Design review of the part built by this model. Coordinates are the model's own, in mm. A direction names the side the tool comes from. Coordinates: 2 decimals unless noted, no trailing zeros. Loops run counter-clockwise (first coordinate to the right, second up) from the corner with the lowest first, then second, coordinate; pieces in that order, holes last. Notation, with made-up numbers: (-35.75, 79) - (-19.75, 79) arc R24 cw to (-19.75, 102) - close; hole circle Ø9 at (30, 56). An arc over 180 degrees is marked (long way). Return JSON: item names as keys, results as strings. Group by question number.
from build123d import *

# Parameters (mm, degrees)
BOSS_EXTRUDE1_DEPTH = 2
SKETCH4_R           = 1.6
CUT_EXTRUDE4_DEPTH  = 414.677410551
SKETCH3_R           = 2.5
SKETCH3_R_2         = 1.5
BOSS_EXTRUDE3_DEPTH = 1
SKETCH5_W           = 24
SKETCH5_H           = 28
BOSS_EXTRUDE2_DEPTH = 7
SKETCH2_W           = 19
SKETCH2_H           = 24.51763809
CUT_EXTRUDE5_DEPTH  = 9
BOSS_EXTRUDE4_REACH = 375.267
SKETCH8_W           = 28
SKETCH8_H           = 24
SKETCH9_R           = 1.5
CUT_EXTRUDE7_DEPTH  = 414.770467772


with BuildPart() as part:
    # Sketch1 → Boss-Extrude1 (new body)
    with BuildSketch(Plane.XY):
        with BuildLine():
            Line((0, 2), (288, 2))
            ThreePointArc((288, 2), (289.414213562, 1.414213562), (290, 0))
            Line((290, 0), (290, -293))
            ThreePointArc((290, -293), (289.414213562, -294.414213562), (288, -295))
            Line((288, -295), (0, -295))
            ThreePointArc((0, -295), (-1.414213562, -294.414213562), (-2, -293))
            Line((-2, -293), (-2, 0))
            ThreePointArc((-2, 0), (-1.414213562, 1.414213562), (0, 2))
        make_face()
    extrude(amount=BOSS_EXTRUDE1_DEPTH)

    # Sketch4 → Cut-Extrude4 (cut, through all)
    with BuildSketch(Plane(origin=(0, 0, 0), x_dir=(-1, 0, 0), z_dir=(0, 0, -1))):
        with Locations((-271, -256)):
            Circle(SKETCH4_R)
        with Locations(Location((-271, -37, 0), (0, 0, 180))):
            Circle(SKETCH4_R)
        with Locations(Location((-17, -256, 0), (0, 0, 180))):
            Circle(SKETCH4_R)
        with Locations((-17, -37)):
            Circle(SKETCH4_R)
    extrude(amount=-CUT_EXTRUDE4_DEPTH, mode=Mode.SUBTRACT)

    # Sketch3 → Boss-Extrude3 (add)
    # profile 1 of 4: a face of its own
    with BuildSketch(Plane(origin=(0, 0, 2), x_dir=(-1, 0, 0), z_dir=(0, 0, -1))):
        with Locations((-271, -37)):
            Circle(SKETCH3_R)
        with Locations((-271, -37)):
            Circle(SKETCH3_R_2, mode=Mode.SUBTRACT)
    # profile 2 of 4: a face of its own
    with BuildSketch(Plane(origin=(0, 0, 2), x_dir=(-1, 0, 0), z_dir=(0, 0, -1))):
        with Locations(Location((-17, -37, 0), (0, 0, 180))):
            Circle(SKETCH3_R)
        with Locations(Location((-17, -37, 0), (0, 0, 180))):
            Circle(SKETCH3_R_2, mode=Mode.SUBTRACT)
    # profile 3 of 4: a face of its own
    with BuildSketch(Plane(origin=(0, 0, 2), x_dir=(-1, 0, 0), z_dir=(0, 0, -1))):
        with Locations((-17, -256)):
            Circle(SKETCH3_R)
        with Locations((-17, -256)):
            Circle(SKETCH3_R_2, mode=Mode.SUBTRACT)
    # profile 4 of 4: a face of its own
    with BuildSketch(Plane(origin=(0, 0, 2), x_dir=(-1, 0, 0), z_dir=(0, 0, -1))):
        with Locations(Location((-271, -256, 0), (0, 0, 180))):
            Circle(SKETCH3_R)
        with Locations(Location((-271, -256, 0), (0, 0, 180))):
            Circle(SKETCH3_R_2, mode=Mode.SUBTRACT)
    extrude(amount=-BOSS_EXTRUDE3_DEPTH)

    # Sketch5 → Boss-Extrude2 (add)
    with BuildSketch(Plane.XY.offset(2)):
        with Locations((273, -68.5)):
            Rectangle(SKETCH5_W, SKETCH5_H)
        with Locations((273, -224.5)):
            Rectangle(SKETCH5_W, SKETCH5_H)
    extrude(amount=BOSS_EXTRUDE2_DEPTH)

    # Sketch2 → Cut-Extrude5 (cut)
    with BuildSketch(Plane(origin=(19.360490202, 0, -72.51763809), x_dir=(0, -1, 0), z_dir=(-0.25881904510252135, 0, 0.9659258262890681))):
        Polygon((234, 285.704276061), (215, 285.704276061), (215.5, 261.186637971), (233.5, 261.186637971), align=None)
        with Locations((68.5, 273.445457016)):
            Rectangle(SKETCH2_W, SKETCH2_H)
    extrude(amount=CUT_EXTRUDE5_DEPTH, mode=Mode.SUBTRACT)

    # Sketch8 → Boss-Extrude4 (add, up to next)
    with BuildSketch(Plane(origin=(103.407277926, 0, -123.235994969), x_dir=(0, -1, 0), z_dir=(-0.6427876096865406, 0, 0.7660444431189771)), mode=Mode.PRIVATE) as boss_extrude4_sk1:
        with Locations((68.5, 193.722688141)):
            Rectangle(SKETCH8_W, SKETCH8_H)
    boss_extrude4_tool1 = extrude(boss_extrude4_sk1.sketch, amount=-BOSS_EXTRUDE4_REACH, mode=Mode.PRIVATE) - part.part
    # Sketch8 → Boss-Extrude4 (add, up to next)
    with BuildSketch(Plane(origin=(103.407277926, 0, -123.235994969), x_dir=(0, -1, 0), z_dir=(-0.6427876096865406, 0, 0.7660444431189771)), mode=Mode.PRIVATE) as boss_extrude4_sk2:
        with Locations((224.5, 193.722688141)):
            Rectangle(SKETCH8_W, SKETCH8_H)
    boss_extrude4_tool2 = extrude(boss_extrude4_sk2.sketch, amount=-BOSS_EXTRUDE4_REACH, mode=Mode.PRIVATE) - part.part
    add(boss_extrude4_tool1.solids().sort_by_distance((251.807467, -68.5, 1.286549))[0])
    add(boss_extrude4_tool2.solids().sort_by_distance((251.807467, -224.5, 1.286549))[0])

    # Sketch9 → Cut-Extrude7 (cut, through all)
    with BuildSketch(Plane(origin=(0, 0, 0), x_dir=(-1, 0, 0), z_dir=(0, 0, -1))):
        with Locations((-126, -196.5)):
            Circle(SKETCH9_R)
        with Locations((-126, -96.5)):
            Circle(SKETCH9_R)
        with Locations((-22, -96.5)):
            Circle(SKETCH9_R)
        with Locations((-22, -196.5)):
            Circle(SKETCH9_R)
    extrude(amount=-CUT_EXTRUDE7_DEPTH, mode=Mode.SUBTRACT)


solid = part.part
Item 1: Add section B-B (y = -104). State the section outline as (x, z) points, then the cut area to 3 significant figures.
Item 2: Draft analysis for pull direction Z (two halves, no side actions). For faces 4 (the face through (271, -82.5, 5)), 5 (the face through (256.89, -68.3, 5.55)), 6 (the face through (146, -144, 0)), state which applies: pulls with the +Z half, pulls with the -Z half, needs draft (parallel to the pull), parting line crosses it, or undercut.
Item 3: For faces 1 (the face through (256.89, -224.3, 5.55)), 2 (the face through (271, -210.5, 5)), 3 (the face through (285, -71.8, 8.6)), list the 3-axis set-ups (+Z, -Z, +X, -X, +Y, -Y) from which the entire face can be reached by the end or side of a thin tool; tool diameter is ignored.
Item 4: To check wall thickness, follow line 1 (X direction, y = -96.5, z = 0.65); line 2 (Y direction, x = 22, z = 1.05); line 3 (Y direction, x = 271, z = 0.9). State the ranges of each line that lie inside material, in increasing order. Write a range as from..to.
Item 5: Add section C-C (x = 168). State the section outline as (y, z) points.
Item 6: Add section A-A (z = 6.5). State the section outline as (x, y) points (3 decimals), then the cut area to 3 significant figures.
Item 7: For P1, Ø3.5, axis at x = 126, y = -96.5, coming from the -Z side; P2, Ø1.5, axis at x = 121.5, y = -166.5, coming from the +Z side; P3, Ø1.9, axis at x = 271, y = -37, coming from the +Z side; P4, Ø5.5, axis at x = 17, y = -37.5, coming from the +Z side, all flat-tipped, find the tip position at first contact; note any pin that passes through.
Answers below:
{
 "1": {"outline": "(-2, 0) - (290, 0) - (290, 2) - (-2, 2) - close", "area": "584 mm^2"},
 "2": {"face 4": "needs draft", "face 5": "pulls with the +Z half", "face 6": "pulls with the -Z half"},
 "3": {"face 1": "+Z, -X, +Y, -Y", "face 2": "+Z, +X, -X", "face 3": "+Z, +X, +Y, -Y"},
 "4": {"line 1": "x = -2..20.5, 23.5..124.5, 127.5..290", "line 2": "y = -295..-198, -195..-98, -95..2", "line 3": "y = -295..-257.6, -254.4..-233.52, -215.48..-78, -59..-38.6, -35.4..2"},
 "5": {"outline": "(-295, 0) - (2, 0) - (2, 2) - (-295, 2) - close"},
 "6": {"outline": "(258.021, -238.5) - (285, -238.5) - (285, -233.823) - (279.485, -233.715) - (279.485, -215.285) - (285, -215.177) - (285, -210.5) - (258.021, -210.5) - close; (258.021, -82.5) - (285, -82.5) - (285, -78) - (279.485, -78) - (279.485, -59) - (285, -59) - (285, -54.5) - (258.021, -54.5) - close", "area": "1,300 mm^2"},
 "7": {"P1": "stops at z = 0", "P2": "stops at z = 2", "P3": "passes through", "P4": "stops at z = 3"}
}
